```python
from build123d import *

# Parameters (mm, degrees)
SKETCH1_W           = 104
SKETCH1_H           = 104
BOSS_EXTRUDE1_DEPTH = 57.5
BOSS_EXTRUDE1_TAPER = 23
SKETCH2_R           = 25
CUT_EXTRUDE1_DEPTH  = 187.70029459
SKETCH3_R           = 35
SKETCH3_R_2         = 25
CUT_EXTRUDE2_DEPTH  = 10
CUT_EXTRUDE3_START  = -10
SKETCH4_R           = 35
CUT_EXTRUDE3_DEPTH  = 10
SKETCH5_W           = 52
SKETCH5_H           = 52
CUT_EXTRUDE4_DEPTH  = 187.70029459
FILLET1_R           = 15
BOSS_EXTRUDE2_DEPTH = 10
CUT_EXTRUDE5_DEPTH  = 10
FILLET2_R           = 5


with BuildPart() as part:
    # Sketch1 → Boss-Extrude1 (new body)
    with BuildSketch(Plane.XY):
        with Locations((52, 52)):
            Rectangle(SKETCH1_W, SKETCH1_H)
    boss_extrude1 = extrude(amount=BOSS_EXTRUDE1_DEPTH, taper=BOSS_EXTRUDE1_TAPER)

    # Mirror1: Boss-Extrude1 across plane
    add(boss_extrude1.mirror(Plane.XY.offset(57.5)))

    # Sketch2 → Cut-Extrude1 (cut, through all)
    with BuildSketch(Plane.XY.offset(115)):
        with Locations((52, 52)):
            Circle(SKETCH2_R)
    extrude(amount=-CUT_EXTRUDE1_DEPTH, mode=Mode.SUBTRACT)

    # Sketch3 → Cut-Extrude2 (cut)
    with BuildSketch(Plane.XY.offset(115)):
        with Locations((52, 52)):
            Circle(SKETCH3_R)
        with Locations((52, 52)):
            Circle(SKETCH3_R_2, mode=Mode.SUBTRACT)
    extrude(amount=-CUT_EXTRUDE2_DEPTH, mode=Mode.SUBTRACT)

    # Sketch4 → Cut-Extrude3 (cut)
    with BuildSketch(Plane(origin=(0, 0, 0), x_dir=(-1, 0, 0), z_dir=(0, 0, -1)).offset(CUT_EXTRUDE3_START)):
        with Locations(Location((-52, 52, 0), (0, 0, 180))):
            Circle(SKETCH4_R)
    extrude(amount=CUT_EXTRUDE3_DEPTH, mode=Mode.SUBTRACT)

    # Sketch5 → Cut-Extrude4 (cut, through all)
    with BuildSketch(Plane.XY.offset(115)):
        with Locations((78, 26)):
            Rectangle(SKETCH5_W, SKETCH5_H)
    extrude(amount=-CUT_EXTRUDE4_DEPTH, mode=Mode.SUBTRACT)

    # Fillet1
    fillet1_edges = [part.edges().sort_by_distance(p)[0] for p in [
        (52, 79.592698068, 57.5),
        (24.407301932, 52, 57.5),
        (79.592698068, 65.796349034, 57.5),
        (38.203650966, 24.407301932, 57.5),
    ]]
    fillet(fillet1_edges, radius=FILLET1_R)

    # Sketch6 → Boss-Extrude2 (add)
    with BuildSketch(Plane.XY.offset(115)):
        Polygon((52, 0), (52, 3), (3, 3), (3, 101), (101, 101), (101, 52), (104, 52), (104, 104), (0, 104), (0, 0), align=None)
    extrude(amount=BOSS_EXTRUDE2_DEPTH)

    # Sketch7 → Cut-Extrude5 (cut)
    with BuildSketch(Plane.XY.offset(115)):
        with BuildLine():
            Line((10.251025223, 89.50633409), (14.587037586, 85.170321726))
            ThreePointArc((14.587037586, 85.170321726), (16.644660941, 87.355339059), (18.829678274, 89.412962414))
            Line((18.829678274, 89.412962414), (14.49366591, 93.748974777))
            ThreePointArc((14.49366591, 93.748974777), (10.251025223, 93.748974777), (10.251025223, 89.50633409))
        make_face()
        with BuildLine():
            Line((14.587037586, 85.170321726), (18.795655971, 80.961703342))
            ThreePointArc((18.795655971, 80.961703342), (23.038296658, 80.961703342), (23.038296658, 85.204344029))
            Line((23.038296658, 85.204344029), (18.829678274, 89.412962414))
            ThreePointArc((18.829678274, 89.412962414), (16.644660941, 87.355339059), (14.587037586, 85.170321726))
        make_face()
        with BuildLine():
            ThreePointArc((18.829678274, 14.587037586), (16.644660941, 16.644660941), (14.587037586, 18.829678274))
            Line((14.587037586, 18.829678274), (10.251025223, 14.49366591))
            ThreePointArc((10.251025223, 14.49366591), (10.251025223, 10.251025223), (14.49366591, 10.251025223))
            Line((14.49366591, 10.251025223), (18.829678274, 14.587037586))
        make_face()
        with BuildLine():
            Line((18.795655971, 23.038296658), (14.587037586, 18.829678274))
            ThreePointArc((14.587037586, 18.829678274), (16.644660941, 16.644660941), (18.829678274, 14.587037586))
            Line((18.829678274, 14.587037586), (23.038296658, 18.795655971))
            ThreePointArc((23.038296658, 18.795655971), (23.038296658, 23.038296658), (18.795655971, 23.038296658))
        make_face()
        with BuildLine():
            ThreePointArc((89.412962414, 85.170321726), (87.355339059, 87.355339059), (85.170321726, 89.412962414))
            Line((85.170321726, 89.412962414), (80.961703342, 85.204344029))
            ThreePointArc((80.961703342, 85.204344029), (80.961703342, 80.961703342), (85.204344029, 80.961703342))
            Line((85.204344029, 80.961703342), (89.412962414, 85.170321726))
        make_face()
        with BuildLine():
            Line((89.50633409, 93.748974777), (85.170321726, 89.412962414))
            ThreePointArc((85.170321726, 89.412962414), (87.355339059, 87.355339059), (89.412962414, 85.170321726))
            Line((89.412962414, 85.170321726), (93.748974777, 89.50633409))
            ThreePointArc((93.748974777, 89.50633409), (93.748974777, 93.748974777), (89.50633409, 93.748974777))
        make_face()
    extrude(amount=-CUT_EXTRUDE5_DEPTH, mode=Mode.SUBTRACT)

    # Fillet2
    fillet2_edges = [part.edges().sort_by_distance(p)[0] for p in [
        (0, 52, 115),
        (26, 0, 115),
        (52, 104, 115),
        (104, 78, 115),
    ]]
    fillet(fillet2_edges, radius=FILLET2_R)


solid = part.part
```
Here's how the part is built. I have some questions about the finished solid (model axes, mm). A direction names the side the tool comes from. Round coordinates to 2 decimals unless told otherwise and drop trailing zeros. Write each loop counter-clockwise with the first axis right and the second up, starting at its lowest first coordinate (ties: lowest second). Pieces come first, ordered by that corner, then holes.
Q1. Which directions (+Z, -Z, +X, -X, +Y, -Y) give clear straight access to the entire face, cutting with the end or side of a thin tool? Please do faces 1 (the flat face through (81, 52, 62)), 2 (the flat face through (32.142, 10.806, 25.458)), 3 (the flat face through (51.272, 93.194, 25.458)), 4 (the flat face through (17, 87, 105)).
Q2. If we mould it in two halves opening along X, with no side actions, what happens to faces 5 (the flat face through (28, 3, 120)), 6 (the flat face through (52, 25, 62)), 7 (the cylindrical face through (80.916, 81.009, 110.07)), 8 (the flat face through (101, 77, 120))? For each: +X half, -X half, draft (parallel to the pull), parting line (faces both ways), or undercut.
Q3. Please list where these lines run through material, in increasing order: probe 1 along Z at (x, y) = (25.5, 37); probe 2 along Z at (x, y) = (15, 19.5); probe 3 along Z at (x, y) = (90, 95.5).
Q4. If we section it at A-A on y = 70.5: Write out the boundary of the cut face in (x, z).
Q5. If we section it at C-C on z = 85: Write out the boundary of the cut face in (x, y).
Q6. Will these pins go through, and if not, where does the flat tip stop? P1, Ø5, axis at y = 32.5, z = 119.5, coming from the +X side; P2, Ø12, axis at x = 39, z = 65, coming from the -Y side; P3, Ø1, axis at x = 26.5, y = 69.5, coming from the -Z side; P4, Ø5, axis at y = 81, z = 121.5, coming from the -X side.
Q7. If we section it at D-D on y = 41: Write out the boundary of the cut face in (x, z).
Q8. If we section it at B-B on x = 58.5: Write out the boundary of the cut face in (y, z).
Answer below:
1. face 1: +Z, -Z, +X, -Y
1. face 2: +X, -X, -Y
1. face 3: +X, -X, +Y
1. face 4: +Z
2. face 5: draft
2. face 6: +X half
2. face 7: undercut
2. face 8: undercut
3. probe 1: z = 10 to 105
3. probe 2: z = 0 to 35.34, 79.66 to 115
3. probe 3: z = 0 to 20.02, 94.98 to 115
4. outline: (0, 0) - (22.29, 0) - (22.29, 10) - (35.18, 10) - (35.18, 105) - (22.29, 105) - (22.29, 115) - (3, 115) - (3, 125) - (0, 125) - (0, 116.02) arc R5 ccw to (0.4, 114.06) - (21.92, 63.36) arc R15 cw to (21.92, 51.64) - close; (68.82, 10) - (81.71, 10) - (81.71, 0) - (104, 0) - (82.08, 51.64) arc R15 cw to (82.08, 63.36) - (103.6, 114.06) arc R5 ccw to (104, 116.02) - (104, 125) - (101, 125) - (101, 115) - (81.71, 115) - (81.71, 105) - (68.82, 105) - close
5. outline: (12.73, 12.73) - (52, 12.73) - (52, 27) arc R25 cw (long way) to (77, 52) - (91.27, 52) - (91.27, 91.27) - (12.73, 91.27) - close
6. P1: stops at x = 3
6. P2: stops at y = 18.68
6. P3: stops at z = 10
6. P4: stops at x = 0
7. outline: (0, 0) - (18.77, 0) - (18.77, 10) - (29.55, 10) - (29.55, 105) - (18.77, 105) - (18.77, 115) - (3, 115) - (3, 125) - (0, 125) - (0, 116.02) arc R5 ccw to (0.4, 114.06) - (21.92, 63.36) arc R15 cw to (21.92, 51.64) - close
8. outline: (76.14, 10) - (86.39, 10) - (86.39, 0) - (104, 0) - (82.08, 51.64) arc R15 cw to (82.08, 63.36) - (103.6, 114.06) arc R5 ccw to (104, 116.02) - (104, 125) - (101, 125) - (101, 115) - (86.39, 115) - (86.39, 105) - (76.14, 105) - close
